from build123d import *

# Parameters (mm, degrees)
SKETCH1_W           = 30
SKETCH1_H           = 15
SKETCH1_R           = 1.6
BOSS_EXTRUDE1_DEPTH = 5
SKETCH2_W           = 5
SKETCH2_H           = 15
BOSS_EXTRUDE2_DEPTH = 25
CUT_EXTRUDE1_REACH  = 41.765
SKETCH3_R           = 1.6
FILLET1_R           = 25
CUT_EXTRUDE2_START  = -5
SKETCH4_R           = 4.5
CUT_EXTRUDE2_DEPTH  = 39.084220006
CUT_EXTRUDE3_START  = -5
SKETCH5_R           = 4.5
CUT_EXTRUDE3_DEPTH  = 30.369317865


with BuildPart() as part:
    # Sketch1 → Boss-Extrude1 (new body)
    with BuildSketch(Plane.XY):
        Rectangle(SKETCH1_W, SKETCH1_H)
        with Locations((3.4, 0)):
            Circle(SKETCH1_R, mode=Mode.SUBTRACT)
    extrude(amount=BOSS_EXTRUDE1_DEPTH)

    # Sketch2 → Boss-Extrude2 (add)
    with BuildSketch(Plane.XY.offset(5)):
        with Locations((-12.5, 0)):
            Rectangle(SKETCH2_W, SKETCH2_H)
    extrude(amount=BOSS_EXTRUDE2_DEPTH)

    # Sketch3 → Cut-Extrude1 (cut, up to next)
    with BuildSketch(Plane(origin=(-10, 0, 0), x_dir=(0, 0, -1), z_dir=(1, 0, 0)), mode=Mode.PRIVATE) as cut_extrude1_sk1:
        with Locations(Location((-18.4, 0, 0), (0, 0, 90))):
            Circle(SKETCH3_R)
    cut_extrude1_tool1 = extrude(cut_extrude1_sk1.sketch, amount=-CUT_EXTRUDE1_REACH, mode=Mode.PRIVATE) & part.part
    add(cut_extrude1_tool1.solids().sort_by_distance((-10, 0, 18.4))[0], mode=Mode.SUBTRACT)

    # Fillet1
    # the kernel refuses this fillet: 25 mm, written as the material it adds along each edge
    with BuildSketch(Plane(origin=(-10, 7.5, 5), x_dir=(0, 0, 1), z_dir=(0, -1, 0))) as fillet1_piece_1_section:
        with BuildLine():
            CenterArc((FILLET1_R, -FILLET1_R), FILLET1_R, 90, 90)
            Line((0, -FILLET1_R), (0, 0))
            Line((0, 0), (FILLET1_R, 0))
        make_face()
    fillet1_piece_1 = extrude(amount=15, mode=Mode.PRIVATE)
    fillet1_piece_1 = fillet1_piece_1 - Plane(origin=(-4.377200925, 0, 18.4), x_dir=(0, 1, 0), z_dir=(1, 0, 0)) * Cylinder(1.6, 130, mode=Mode.PRIVATE)
    fillet1_piece_1 = fillet1_piece_1 - Plane(origin=(3.4, 0, 10.622848357), x_dir=(1, 0, 0), z_dir=(0, 0, -1)) * Cylinder(1.6, 130, mode=Mode.PRIVATE)
    add(fillet1_piece_1)

    # Sketch4 → Cut-Extrude2 (cut, through all)
    with BuildSketch(Plane.ZY.offset(15).offset(CUT_EXTRUDE2_START)):
        with Locations((18.4, 0)):
            Circle(SKETCH4_R)
    extrude(amount=-CUT_EXTRUDE2_DEPTH, mode=Mode.SUBTRACT)

    # Sketch5 → Cut-Extrude3 (cut, through all)
    with BuildSketch(Plane(origin=(0, 0, 0), x_dir=(-1, 0, 0), z_dir=(0, 0, -1)).offset(CUT_EXTRUDE3_START)):
        with Locations((-3.4, 0)):
            Circle(SKETCH5_R)
    extrude(amount=-CUT_EXTRUDE3_DEPTH, mode=Mode.SUBTRACT)


solid = part.part
Can you work these out from the model? Positions are in its coordinate system, mm. A direction names the side the tool comes from. Round coordinates to 2 decimals unless told otherwise and drop trailing zeros. Loops run counter-clockwise (first coordinate to the right, second up) from the corner with the lowest first, then second, coordinate; pieces in that order, holes last. Notation, with made-up numbers: (36.25, 56.5) - (80.25, 56.5) arc R26 cw to (80.25, 80.5) - close; hole circle Ø3 at (3, -28.75). An arc over 180 degrees is marked (long way). Use CSV: the item, a comma, the result in double quotes. Start each with the question number.
1) We'd pull the mould along Z, two halves only. Please class faces 1 (the flat face through (-10, -2, 18)), 2 (the cylindrical face through (-7.736, 0.198, 13.904)), 3 (the flat face through (0, 0, 0)), 4 (the cylindrical face through (5, 0, 2)): released by +Z, released by -Z, zero draft, split by the parting line, or undercut.
2) If we section it at A-A on x = -11: Write out the boundary of the cut face in (y, z).
3) If we section it at B-B on y = 0.5: Write out the boundary of the cut face in (x, z).
4) For faces 5 (the flat face through (-15, 0, 15)), 6 (the cylindrical face through (-0.892, 1.352, 7.243)), which set-ups out of +Z, -Z, +X, -X, +Y, -Y let a thin tool reach every point of the face, with its end or its side?
5) If we section it at C-C on x = 3.4: Write out the boundary of the cut face in (y, z), plus the area to 3 significant figures.
6) Please list where these lines run through material, in increasing order: probe 1 along X at (y, z) = (0, 1.45); probe 2 along Y at (x, z) = (-8.15, 18.4); probe 3 along Z at (x, y) = (-13.95, 0). Write a range as [from, to].
7) If we section it at D-D on z = 18.4: Write out the boundary of the cut face in (x, y).
8) For pin 1 Ø5 at (y, z) = (0, 18.4) entering from +X; pin 2 Ø7 at (x, y) = (3.4, 0) entering from -Z; pin 3 Ø4.5 at (x, y) = (4, 2) entering from +Z; pin 4 Ø8 at (x, y) = (0, 2) entering from +Z, each with a flat end and sliding along its axis, tell me the tip position at first contact or that it passes through.
Geometry results:
1,face 1,"undercut"
1,face 2,"undercut"
1,face 3,"released by -Z"
1,face 4,"zero draft"
2,outline,"(-7.5, 0) - (7.5, 0) - (7.5, 30) - (-7.5, 30) - close; hole circle Ø3.2 at (0, 18.4)"
3,outline,"(-15, 0) - (1.88, 0) - (1.88, 5) - (-1.07, 5) - (-1.07, 10.85) arc R25 cw to (-4.15, 13.93) - (-10, 13.93) - (-10, 16.88) - (-15, 16.88) - close; (-15, 19.92) - (-10, 19.92) - (-10, 22.87) - (-8.96, 22.87) arc R25 cw to (-10, 30) - (-15, 30) - close; (4.92, 0) - (15, 0) - (15, 5) arc R25 cw to (7.87, 6.04) - (7.87, 5) - (4.92, 5) - close"
4,face 5,"+Z, -Z, -X, +Y, -Y"
4,face 6,"+Z"
5,outline,"(-7.5, 0) - (-1.6, 0) - (-1.6, 5) - (-4.5, 5) - (-4.5, 7.85) - (-7.5, 7.85) - close; (1.6, 0) - (7.5, 0) - (7.5, 7.85) - (4.5, 7.85) - (4.5, 5) - (1.6, 5) - close"
5,area,"76.1 mm2"
6,probe 1,"x = [-15, 1.8], [5, 15]"
6,probe 2,"y = [-7.5, -4.5], [4.5, 7.5]"
6,probe 3,"z = [0, 16.8], [20, 30]"
7,outline,"(-15, -7.5) - (-7.15, -7.5) - (-7.15, -4.5) - (-10, -4.5) - (-10, -1.6) - (-15, -1.6) - close; (-15, 1.6) - (-10, 1.6) - (-10, 4.5) - (-7.15, 4.5) - (-7.15, 7.5) - (-15, 7.5) - close"
8,pin 1,"stops at x = -10"
8,pin 2,"stops at z = 0"
8,pin 3,"stops at z = 5"
8,pin 4,"stops at z = 13.75"
